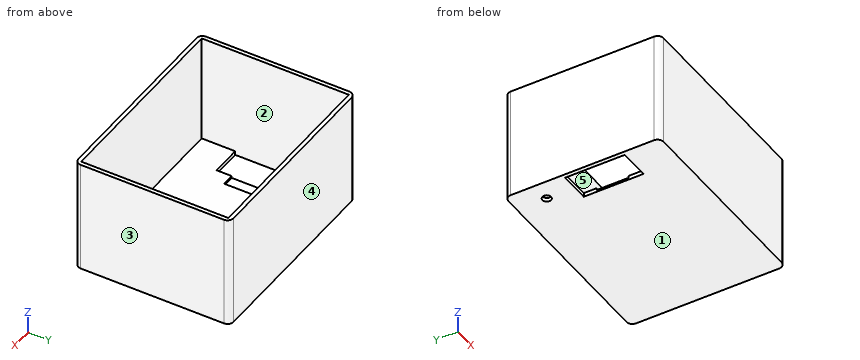
from build123d import *

# Parameters (mm, degrees)
F0_W     = 78
F0_H     = 57
F1_DEPTH = 103
F2_T     = -2
F3_W     = 15.3
F3_H     = 30
F4_DEPTH = 2
F5_W     = 6.151636
F5_H     = 16.015052
F6_DEPTH = 1
F7_R     = 3
F8_R     = 2.19301
F9_DEPTH = 25


with BuildPart() as f1:
    # F0 (on Right) → F1 (new body)
    with BuildSketch(Plane.YZ):
        with Locations((2.376287, -1.899485)):
            Rectangle(F0_W, F0_H)
    extrude(amount=F1_DEPTH)

    # F2
    f2_openings = [f1.faces().sort_by_distance(p)[0] for p in [
        (51.5, 2.376287, 26.600515),
    ]]
    offset(amount=F2_T, openings=f2_openings)

    # F3 (on face) → F4 (cut)
    with BuildSketch(Plane.XY.offset(-28.399485)):
        with Locations((9.65, -2.759746)):
            Rectangle(F3_W, F3_H)
    extrude(amount=-F4_DEPTH, mode=Mode.SUBTRACT)

    # F5 (on face) → F6 (cut)
    with BuildSketch(Plane.XY.offset(-28.399485)):
        with Locations((20.375818, -2.137607)):
            Rectangle(F5_W, F5_H)
    extrude(amount=-F6_DEPTH, mode=Mode.SUBTRACT)

    # F7
    f7_edges = [f1.edges().sort_by_distance(p)[0] for p in [
        (0, -36.623713, -1.899485),
        (0, 41.376287, -1.899485),
        (103, 41.376287, -1.899485),
        (103, -36.623713, -1.899485),
    ]]
    fillet(f7_edges, radius=F7_R)

    # F8 (on face) → F9 (cut)
    with BuildSketch(Plane(origin=(0, 0, -30.399485), x_dir=(1, 0, 0), z_dir=(0, 0, -1))):
        with Locations((10, -26.376287)):
            Circle(F8_R)
    extrude(amount=-F9_DEPTH, mode=Mode.SUBTRACT)


solid = f1.part
The listing builds one solid part. Answer for the finished solid, in the listing's coordinates (mm). Face numbers are marked on the shaded views. A direction names the side the tool comes from. Give positions to 0.01 mm unless a question says otherwise; leave off trailing zeros. Write each loop counter-clockwise with the first axis right and the second up, starting at its lowest first coordinate (ties: lowest second). Pieces come first, ordered by that corner, then holes. Notation, with made-up numbers: (52.25, -20) -> (77.25, -20) arc R6 ccw to (77.25, -11) -> close; hole circle Ø2 at (-25.5, 61). An arc over 180 degrees is marked (long way). One line per question, with ' | ' between items. Start each with the question number.
1. For the marked faces 1 and 2, determine the directions among +Z, -Z, +X, -X, +Y, -Y from which every point of the face is accessible in a straight line to the end or side of a thin tool.
2. Given pin 1 Ø1.8 at (x, y) = (19, -4.5) entering from +Z; pin 2 Ø2 at (x, y) = (36.5, -24) entering from +Z, each flat-ended and moving along its own axis, determine where each tip first touches the part or whether it passes through.
3. Section C-C (z = -5) is taken. Determine the outline of the cut face in (x, y), plus the area to 3 significant figures.
4. Find the intervals of material crossed by probe 1 along X at (y, z) = (-20, 11); probe 2 along Y at (x, z) = (69.5, 24.5); probe 3 along Y at (x, z) = (10, -29), in increasing order.
5. For a pull along Y with two mould halves and no side action, classify the marked faces 3, 4 and 5 as pulls with the +Y half, pulls with the -Y half, needs draft (parallel to the pull), parting line crosses it, or undercut.
6. Section A-A (x = 10) is taken. Determine the outline of the cut face in (y, z), plus the area to 3 significant figures.
7. Section D-D (x = 72) is taken. Determine the outline of the cut face in (y, z), plus the area to 3 significant figures.
8. Section B-B (y = 7) is taken. Determine the outline of the cut face in (x, z).
Response values:
1) face 1: -Z, +X, -X, +Y, -Y | face 2: +Z
2) pin 1: z = -29.4 | pin 2: z = -28.4
3) outline: (0, -33.62) arc R3 ccw to (3, -36.62) -> (100, -36.62) arc R3 ccw to (103, -33.62) -> (103, 38.38) arc R3 ccw to (100, 41.38) -> (3, 41.38) arc R3 ccw to (0, 38.38) -> close; hole (2, -34.62) -> (101, -34.62) -> (101, 39.38) -> (2, 39.38) -> close | area: 700 mm2
4) probe 1: 0 to 2, 101 to 103 | probe 2: -36.62 to -34.62, 39.38 to 41.38 | probe 3: -36.62 to -17.76, 12.24 to 24.18, 28.57 to 41.38
5) face 3: needs draft | face 4: pulls with the +Y half | face 5: undercut
6) outline: (-36.62, -30.4) -> (-17.76, -30.4) -> (-17.76, -28.4) -> (-34.62, -28.4) -> (-34.62, 26.6) -> (-36.62, 26.6) -> close; (12.24, -30.4) -> (24.18, -30.4) -> (24.18, -28.4) -> (12.24, -28.4) -> close; (28.57, -30.4) -> (41.38, -30.4) -> (41.38, 26.6) -> (39.38, 26.6) -> (39.38, -28.4) -> (28.57, -28.4) -> close | area: 307 mm2
7) outline: (-36.62, -30.4) -> (41.38, -30.4) -> (41.38, 26.6) -> (39.38, 26.6) -> (39.38, -28.4) -> (-34.62, -28.4) -> (-34.62, 26.6) -> (-36.62, 26.6) -> close | area: 376 mm2
8) outline: (0, -30.4) -> (2, -30.4) -> (2, 26.6) -> (0, 26.6) -> close; (17.3, -30.4) -> (103, -30.4) -> (103, 26.6) -> (101, 26.6) -> (101, -28.4) -> (17.3, -28.4) -> close
